Model file for the job. Use its own axes, mm. A direction names the side the tool comes from. Coordinates: 2 decimals unless noted, no trailing zeros. Loops run counter-clockwise (first coordinate to the right, second up) from the corner with the lowest first, then second, coordinate; pieces in that order, holes last. Notation, with made-up numbers: (-4, -18.5) -> (17, -18.5) arc R21 ccw to (17, 1.5) -> close; hole circle Ø8 at (9.5, 18). An arc over 180 degrees is marked (long way). Use one line per item in the form item = value.
```python
from build123d import *

# Parameters (mm, degrees)
SKETCH1_R           = 9.25
SKETCH1_R_2         = 3
BOSS_EXTRUDE1_DEPTH = 19
SKETCH2_OUTSIDE_W   = 26.966
SKETCH2_OUTSIDE_H   = 26.966
SKETCH2_OUTSIDE_R   = 4.5
CUT_EXTRUDE1_DEPTH  = 6.5
SKETCH3_OUTSIDE_W   = 26.966
SKETCH3_OUTSIDE_H   = 26.966
SKETCH3_OUTSIDE_R   = 6.8
CUT_EXTRUDE2_DEPTH  = 8.5
SKETCH4_OUTSIDE_W   = 26.966
SKETCH4_OUTSIDE_H   = 26.966
SKETCH4_OUTSIDE_R   = 6.55
CUT_EXTRUDE3_DEPTH  = 7
CHAMFER1_SIZE       = 0.5
CUT_EXTRUDE4_START  = -5
SKETCH5_OUTSIDE_W   = 26.966
SKETCH5_OUTSIDE_H   = 26.966
SKETCH5_OUTSIDE_R   = 6
CUT_EXTRUDE4_DEPTH  = 2


with BuildPart() as part:
    # Sketch1 → Boss-Extrude1 (new body)
    with BuildSketch(Plane.XY):
        Circle(SKETCH1_R)
        Circle(SKETCH1_R_2, mode=Mode.SUBTRACT)
    extrude(amount=BOSS_EXTRUDE1_DEPTH)

    # Sketch2 outside → Cut-Extrude1 (cut)
    with BuildSketch(Plane.XY.offset(19)):
        Rectangle(SKETCH2_OUTSIDE_W, SKETCH2_OUTSIDE_H)
        Circle(SKETCH2_OUTSIDE_R, mode=Mode.SUBTRACT)
    extrude(amount=-CUT_EXTRUDE1_DEPTH, mode=Mode.SUBTRACT)

    # Sketch3 outside → Cut-Extrude2 (cut)
    with BuildSketch(Plane(origin=(0, 0, 0), x_dir=(-1, 0, 0), z_dir=(0, 0, -1))):
        Rectangle(SKETCH3_OUTSIDE_W, SKETCH3_OUTSIDE_H)
        Circle(SKETCH3_OUTSIDE_R, mode=Mode.SUBTRACT)
    extrude(amount=-CUT_EXTRUDE2_DEPTH, mode=Mode.SUBTRACT)

    # Sketch4 outside → Cut-Extrude3 (cut)
    with BuildSketch(Plane(origin=(0, 0, 0), x_dir=(-1, 0, 0), z_dir=(0, 0, -1))):
        Rectangle(SKETCH4_OUTSIDE_W, SKETCH4_OUTSIDE_H)
        Circle(SKETCH4_OUTSIDE_R, mode=Mode.SUBTRACT)
    extrude(amount=-CUT_EXTRUDE3_DEPTH, mode=Mode.SUBTRACT)

    # Chamfer1
    chamfer1_edges = [part.edges().sort_by_distance(p)[0] for p in [
        (-4.5, 0, 19),
    ]]
    chamfer(chamfer1_edges, length=CHAMFER1_SIZE)

    # Sketch5 outside → Cut-Extrude4 (cut)
    with BuildSketch(Plane(origin=(0, 0, 0), x_dir=(-1, 0, 0), z_dir=(0, 0, -1)).offset(CUT_EXTRUDE4_START)):
        Rectangle(SKETCH5_OUTSIDE_W, SKETCH5_OUTSIDE_H)
        Circle(SKETCH5_OUTSIDE_R, mode=Mode.SUBTRACT)
    extrude(amount=-CUT_EXTRUDE4_DEPTH, mode=Mode.SUBTRACT)


solid = part.part
```
Q1. Pin check, flat tips, straight feed: pin 1 Ø3 at (x, z) = (-3.5, 8) entering from -Y; pin 2 Ø1 at (x, y) = (6, 3.5) entering from +Z; pin 3 Ø1.5 at (x, z) = (2.5, 11.5) entering from +Y. Stop position of each tip, or through.
Result:
pin_1 = -9.01
pin_2 = 12.5
pin_3 = 9.08
Q2. Band-saw the part on A-A, the plane y = 0. Write the cut outline in (x, z).
Result:
outline = (-9.25, 8.5) -> (-6.8, 8.5) -> (-6.8, 7) -> (-6, 7) -> (-6, 5) -> (-6.55, 5) -> (-6.55, 0) -> (-3, 0) -> (-3, 19) -> (-4, 19) -> (-4.5, 18.5) -> (-4.5, 12.5) -> (-9.25, 12.5) -> close; (3, 0) -> (6.55, 0) -> (6.55, 5) -> (6, 5) -> (6, 7) -> (6.8, 7) -> (6.8, 8.5) -> (9.25, 8.5) -> (9.25, 12.5) -> (4.5, 12.5) -> (4.5, 18.5) -> (4, 19) -> (3, 19) -> close
Q3. Which spindle directions (+Z, -Z, +X, -X, +Y, -Y) get a long thin tool onto all of the face, cutting with end or side? Do faces 1 (the face through (1.47, -6.64, 7.74)), 2 (the face through (-0.59, 4.46, 15.54)), 3 (the face through (-6, -2, 5)). Say none if no direction does.
Result:
face_1 = -Z
face_2 = +Z
face_3 = none
Q4. Mould opens along Y. For faces 4 (the face through (-3, 0, 9)), 5 (the face through (0.853, 6.494, 2.465)), 6 (the face through (-4, -5, 7)) say: released by +Y, released by -Y, zero draft, split by the parting line, or undercut.
Result:
face_4 = undercut
face_5 = split by the parting line
face_6 = zero draft
Q5. Band-saw the part on C-C, the plane z = 16.5. Write the cut outline in (x, y).
Result:
outline = circle Ø9 at (0, 0); hole circle Ø6 at (0, 0)
Q6. Wall check: line 1 along Y through (x, z) = (0, 12); line 2 along Y through (x, z) = (0, 6.75); line 3 along Z through (x, y) = (-7, 3.25). Give the ranges that are in metal, low to high.
Result:
line_1 = -9.25 to -3, 3 to 9.25
line_2 = -6 to -3, 3 to 6
line_3 = 8.5 to 12.5
Q7. Band-saw the part on D-D, the plane x = 5.25. Write the cut outline in (y, z).
Result:
outline = (-7.62, 8.5) -> (-4.32, 8.5) -> (-4.32, 7) -> (-2.9, 7) -> (-2.9, 5) -> (-3.92, 5) -> (-3.92, 0) -> (3.92, 0) -> (3.92, 5) -> (2.9, 5) -> (2.9, 7) -> (4.32, 7) -> (4.32, 8.5) -> (7.62, 8.5) -> (7.62, 12.5) -> (-7.62, 12.5) -> close
